Autodesk Inventor part; units mm, degrees
ref_plane "YZ Plane" through (0, 0, 0) normal (1, 0, 0) x (0, 1, 0)
ref_plane "XZ Plane" through (0, 0, 0) normal (0, 1, 0) x (-1, 0, 0)
ref_plane "XY Plane" through (0, 0, 0) normal (0, 0, 1) x (1, 0, 0)
sketch "Sketch1" plane through (0, 0, 0) normal (0, 0, 1) x (1, 0, 0)
  line L0 (0, 0) -> (12.7, 0)
  line L1 (12.7, 0) -> (12.7, 12.7)
  line L2 (12.7, 12.7) -> (0, 12.7)
  line L3 (0, 12.7) -> (0, 0)
  dimension "d0" = 12.7
  dimension "d1" = 12.7
extrude "Extrusion1" add sketch "Sketch1" along normal blind 648.4937
sketch "Sketch2" plane through (12.7, 12.7, 648.4937) normal (0, 1, 0) x (1, 0, 0)
  line L0 (-12.7, 0) -> (0, 0)
  line L1 (0, 648.4937) -> (0, 0)
  line L2 (0, 648.4937) -> (-12.7, 648.4937)
  line L3 (-12.7, 648.4937) -> (-12.7, 0)
  line L4 (-12.7, 15.875) -> (-9.525, 15.875)
  line L5 (-9.525, 15.875) -> (-9.525, 632.6187)
  line L6 (-9.525, 632.6187) -> (-12.7, 632.6187)
  line L7 (-12.7, 632.6187) -> (-12.7, 15.875)
  line L8 (0, 632.6187) -> (-3.175, 632.6187)
  line L9 (-3.175, 632.6187) -> (-3.175, 15.875)
  line L10 (-3.175, 15.875) -> (0, 15.875)
  line L11 (0, 15.875) -> (0, 632.6187)
  line L12 (-9.525, 648.4937) -> (-3.175, 648.4937)
  line L13 (-3.175, 648.4937) -> (-3.175, 635.7937)
  line L14 (-3.175, 635.7937) -> (-9.525, 635.7937)
  line L15 (-9.525, 635.7937) -> (-9.525, 648.4937)
  line L16 (-9.525, 0) -> (-3.175, 0)
  line L17 (-3.175, 0) -> (-3.175, 12.7)
  line L18 (-3.175, 12.7) -> (-9.525, 12.7)
  line L19 (-9.525, 12.7) -> (-9.525, 0)
  dimension "d4" = 15.875
  dimension "d5" = 6.35
  dimension "d6" = 15.875
  dimension "d7" = 12.7
  dimension "d8" = 12.7
extrude "Extrusion2" cut sketch "Sketch2" against normal through all contours L19 L18 L17 L0 | L3 L6 L5 L4 | L10 L9 L8 L1 | L2 L13 L14 L15
sketch "Sketch3" plane through (12.7, 0, 648.4937) normal (1, 0, 0) x (0, 0, -1)
  line L0 (15.875, 12.7) -> (0, 12.7)
  line L1 (0, 12.7) -> (0, 0)
  line L2 (632.6187, 12.7) -> (632.6187, 0)
  line L3 (648.4937, 0) -> (632.6187, 0)
  line L4 (648.4937, 0) -> (648.4937, 12.7)
  line L5 (648.4937, 12.7) -> (632.6187, 12.7)
  line L6 (632.6187, 0) -> (15.875, 0)
  line L7 (632.6187, 12.7) -> (632.6187, 0)
  line L8 (15.875, 12.7) -> (632.6187, 12.7)
  line L9 (15.875, 12.7) -> (15.875, 0)
  line L10 (15.875, 12.7) -> (632.6187, 12.7)
  line L11 (632.6187, 12.7) -> (632.6187, 9.525)
  line L12 (632.6187, 9.525) -> (15.875, 9.525)
  line L13 (15.875, 9.525) -> (15.875, 12.7)
  line L14 (632.6187, 3.175) -> (15.875, 3.175)
  line L15 (15.875, 3.175) -> (15.875, 0)
  line L16 (15.875, 0) -> (632.6187, 0)
  line L17 (632.6187, 0) -> (632.6187, 3.175)
  circle A0 centre (6.35, 6.35) radius 3.175
  circle A1 centre (642.1437, 6.35) radius 3.175
  point P0 (648.4937, 0)
  dimension "d11" = 6.35
  dimension "d12" = 6.35
  dimension "d13" = 6.35
  dimension "d14" = 6.35
  dimension "d15" = 3.175
  dimension "d16" = 6.35
  dimension "d17" = 6.35
  dimension "d18" = 6.35
extrude "Extrusion3" cut sketch "Sketch3" against normal through all contours L2 L12 L9 L8 | L2 L6 L9 L14 | A0 | A1
fillet "Fillet1" radius 3.175 4 edges at (9.525, 9.525, 324.2469) (3.175, 9.525, 324.2469) (3.175, 3.175, 324.2469) (9.525, 3.175, 324.2469)
equation "\"d1\" = d0"
equation "\"d13\" = d12"
equation "\"d17\" = d16"
equation "\"d18\" = d17"
properties part number "manipulator piston"
Here's how the part is built. I have some questions about the finished solid (model axes, mm). A direction names the side the tool comes from. Round coordinates to 2 decimals unless told otherwise and drop trailing zeros. Use CSV: the item, a comma, the result in double quotes.
1) If we mould it in two halves opening along X, with no side actions, what happens to faces 1 (the flat face through (12.7, 6, 10)), 2 (the flat face through (6, 0, 13)), 3 (the flat face through (3.175, 9.3, 640.6))? For each: pulls with the +X half, pulls with the -X half, needs draft (parallel to the pull), parting line crosses it, or undercut.
Taken from the geometry:
face 1,"pulls with the +X half"
face 2,"needs draft"
face 3,"undercut"
2) I need wall thicknesses on line 1 along Z through (x, y) = (10.5, 7.25) (3 decimals); line 2 along Z through (x, y) = (3.75, 1) (3 decimals); line 3 along Y through (x, z) = (10.2, 6.35) (3 decimals). Which ranges of each line are inside material? Lowest first, please. Write a range as [from, to].
Taken from the geometry:
line 1,"[0, 3.305], [9.395, 15.875], [632.619, 639.099], [645.188, 648.494]"
line 2,"[12.7, 15.875], [632.619, 635.794]"
line 3,"[0, 3.175], [9.525, 12.7]"
3) On a 3-axis mill with a long thin cutter (end or side, diameter ignored), from which of +Z, -Z, +X, -X, +Y, -Y can I reach the whole of each face in a straight line? I mean faces 4 (the flat face through (9.525, 9.3, 4.8)), 5 (the flat face through (9.525, 7.9, 645.1)), 6 (the flat face through (4.8, 9.3, 632.619)), 7 (the flat face through (6, 0, 635)), 8 (the flat face through (6, 12.7, 13)). Say none if no direction works.
Taken from the geometry:
face 4,"-Z, +Y, -Y"
face 5,"+Z, +Y, -Y"
face 6,"none"
face 7,"+Z, -Z, +X, -X, -Y"
face 8,"+Z, -Z, +X, -X, +Y"
4) I'm going to push flat-ended pins straight in: P1, Ø5, axis at x = 7, z = 530, coming from the +Y side (3 decimals); P2, Ø3, axis at y = 4.5, z = 102.5, coming from the -X side; P3, Ø1.5, axis at x = 8, y = 10, coming from the +Z side; P4, Ø5, axis at y = 6.35, z = 6.35, coming from the -X side. Where does each tip first touch, or does it pass through?
Taken from the geometry:
P1,"y = 9.525"
P2,"x = 3.19"
P3,"z = 635.79"
P4,"through"
